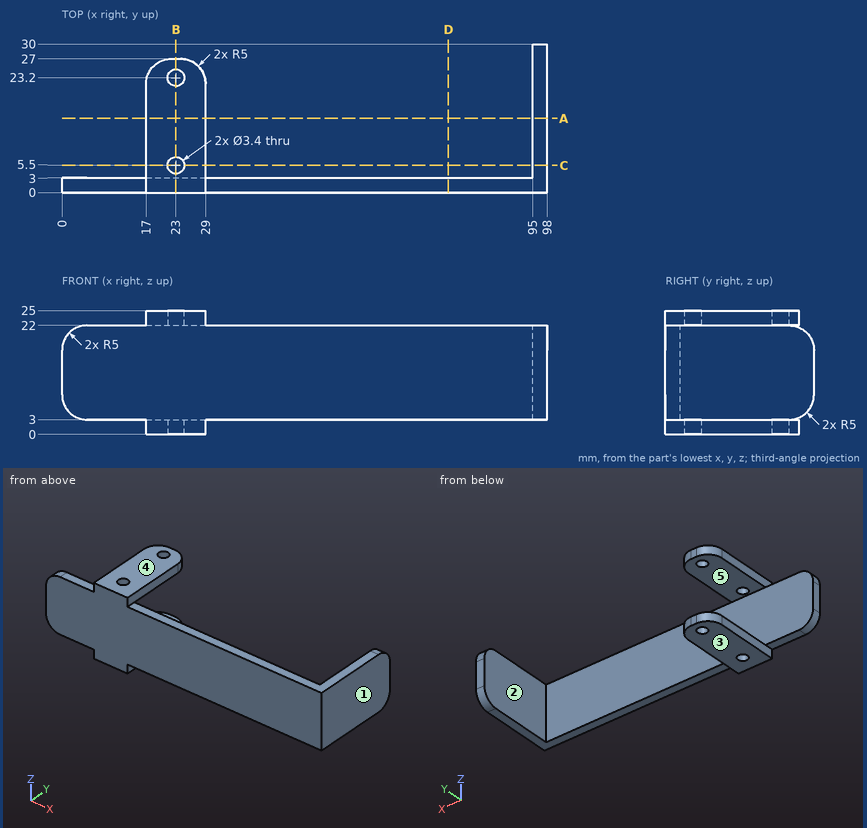
For this review, use the dimensioned drawing (mm, ordinates from the lowest corner) and the shaded views. A direction names the side the tool comes from. Give positions to 0.01 mm unless a question says otherwise; leave off trailing zeros. Loops run counter-clockwise (first coordinate to the right, second up) from the corner with the lowest first, then second, coordinate; pieces in that order, holes last. Notation, with made-up numbers: (12.25, -10) -> (21.25, -10) arc R13 cw to (21.25, -1) -> close; hole circle Ø7 at (-38, -16). An arc over 180 degrees is marked (long way). One line per question, with ' | ' between items. Start each with the question number.
(1) We need section C-C (y = 5.5). State the section outline as (x, z) points.
(2) Draft analysis for pull direction Z (two halves, no side actions). For the marked faces 3, 4 and 5, state which applies: +Z half, -Z half, draft (parallel to the pull), parting line (faces both ways), or undercut.
(3) We need section B-B (x = 23). State the section outline as (y, z) points.
(4) We need section A-A (y = 15). State the section outline as (x, z) points, and give its area (3 significant figures).
(5) Insertion check: P1, Ø10, axis at x = 30.5, z = 11, coming from the +Y side; P2, Ø2.5, axis at x = 23, y = 5.5, coming from the +Z side; P3, Ø0.6, axis at x = 23, z = 1.5, coming from the +Y side; P4, Ø10, axis at x = 61.5, y = 6.5, coming from the +Z side. Each pin has a flat end and moves straight along its axis. Give the tip position at first contact, or say it passes through.
(6) For line 1 (Y direction, x = 23, z = 23.75); line 2 (Z direction, x = 25, y = 23); line 3 (X direction, y = 5.5, z = 23.3), list the stretches that pass through material, from the lowest coordinate up.
(7) For the marked faces 1 and 2, list the 3-axis set-ups (+Z, -Z, +X, -X, +Y, -Y) from which the entire face can be reached by the end or side of a thin tool; tool diameter is ignored.
(8) We need section D-D (x = 78). State the section outline as (y, z) points.
The answers:
1) outline: (17, 0) -> (21.3, 0) -> (21.3, 3) -> (17, 3) -> close; (17, 22) -> (21.3, 22) -> (21.3, 25) -> (17, 25) -> close; (24.7, 0) -> (29, 0) -> (29, 3) -> (24.7, 3) -> close; (24.7, 22) -> (29, 22) -> (29, 25) -> (24.7, 25) -> close; (95, 3) -> (98, 3) -> (98, 22) -> (95, 22) -> close
2) face 3: -Z half | face 4: +Z half | face 5: undercut
3) outline: (0, 0) -> (3.8, 0) -> (3.8, 3) -> (3, 3) -> (3, 22) -> (3.8, 22) -> (3.8, 25) -> (0, 25) -> close; (7.2, 0) -> (21.5, 0) -> (21.5, 3) -> (7.2, 3) -> close; (7.2, 22) -> (21.5, 22) -> (21.5, 25) -> (7.2, 25) -> close; (24.9, 0) -> (27, 0) -> (27, 3) -> (24.9, 3) -> close; (24.9, 22) -> (27, 22) -> (27, 25) -> (24.9, 25) -> close
4) outline: (17, 0) -> (29, 0) -> (29, 3) -> (17, 3) -> close; (17, 22) -> (29, 22) -> (29, 25) -> (17, 25) -> close; (95, 3) -> (98, 3) -> (98, 22) -> (95, 22) -> close | area: 129 mm^2
5) P1: stops at y = 3 | P2: passes through | P3: stops at y = 27 | P4: stops at z = 22
6) line 1: y = 0 to 3.8, 7.2 to 21.5, 24.9 to 27 | line 2: z = 0 to 3, 22 to 25 | line 3: x = 17 to 21.3, 24.7 to 29
7) face 1: +Z, -Z, +X, +Y, -Y | face 2: +Z, -Z, -X, +Y
8) outline: (0, 3) -> (3, 3) -> (3, 22) -> (0, 22) -> close
